Check sheet for the modelled part. Datum: model origin and axes. Units: mm. Face numbers are marked on the shaded views. A direction names the side the tool comes from. Coordinates: 2 decimals unless noted, no trailing zeros. Loops run counter-clockwise (first coordinate to the right, second up) from the corner with the lowest first, then second, coordinate; pieces in that order, holes last. Notation, with made-up numbers: (61.25, -14.75) - (117.25, -14.75) arc R20 cw to (117.25, 22.25) - close; hole circle Ø10 at (-15.5, -23). An arc over 180 degrees is marked (long way). Write each question's results on one line, items separated by ' | '. Start each with the question number.
1. Gauge pin test, flat ends, axial feed: P1, Ø12, axis at y = 31, z = 2.5, coming from the -X side; P2, Ø4, axis at y = 26, z = -18.5, coming from the +X side; P3, Ø6, axis at y = 20, z = 18.5, coming from the +X side; P4, Ø1.5, axis at x = -38.5, y = 20.5, coming from the -Z side. Record the tip position at first contact, or that the pin passes through.
2. Draft check along Z on the marked faces 6, 7, 8 and 9. Enter one of: released by +Z, released by -Z, zero draft, split by the parting line, or undercut.
3. Tool access check on the marked faces 1, 2, 3, 4 and 5. Record the directions out of +Z, -Z, +X, -X, +Y, -Y that give a thin tool (end or side, any length) a straight path to the whole face; none if there is none.
4. Cross-section at C-C (x = -33). Give the number of separate pieces and of enclosed holes in the cut face, and give its area (3 significant figures).
5. Cross-section at A-A (z = -33.5). Record the cut outline in (x, y).
6. Thickness scan on line 1 (Z direction, x = -29.5, y = 29); line 2 (Z direction, x = -17.5, y = 22); line 3 (Y direction, x = -31.5, z = -1). Record the ranges inside material, lowest first. Write a range as [from, to].
7. Cross-section at D-D (z = -15). Record the cut outline in (x, y), and give its area (3 significant figures).
8. Cross-section at B-B (y = 14). Record the cut outline in (x, z), and give its area (3 significant figures).
```python
from build123d import *

# Parameters (mm, degrees)
F0_R      = 8.5
F1_DEPTH  = 32
F4_DEPTH  = 32.4
F5_SIZE   = 1
F6_R      = 15
F7_DEPTH  = 16
F8_R      = 8.5
F9_DEPTH  = 32
F10_SIZE  = 1
F13_DEPTH = 46.1
F15_R     = 6.055959
F16_DEPTH = 53.1


with BuildPart() as f1:
    # F0 (on Top) → F1 (new body)
    with BuildSketch(Plane.XY):
        with Locations((-31.744916, 24.020635)):
            Circle(F0_R)
    extrude(amount=F1_DEPTH)

    # F3 (on offset) → F4 (cut)
    with BuildSketch(Plane.XZ.offset(-33)):
        with BuildLine():
            ThreePointArc((-28.736681, 21.964274), (-31.682465, 24.910059), (-34.62825, 21.964274))
            Line((-34.62825, 21.964274), (-34.62825, 9.964274))
            ThreePointArc((-34.62825, 9.964274), (-31.682465, 7.01849), (-28.736681, 9.964274))
            Line((-28.736681, 9.964274), (-28.736681, 21.964274))
        make_face()
    extrude(amount=F4_DEPTH, mode=Mode.SUBTRACT)

    # F5
    f5_edges = [f1.edges().sort_by_distance(p)[0] for p in [
        (-40.244916, 24.020635, 32),
    ]]
    chamfer(f5_edges, length=F5_SIZE)

    # F6 (on face) → F7 (join)
    with BuildSketch(Plane(origin=(0, 0, 0), x_dir=(1, 0, 0), z_dir=(0, 0, -1))):
        with Locations((-31.744916, -24.020635)):
            Circle(F6_R)
    extrude(amount=F7_DEPTH)

    # F8 (on face) → F9 (join)
    with BuildSketch(Plane(origin=(0, 0, -16), x_dir=(1, 0, 0), z_dir=(0, 0, -1))):
        with Locations((-31.744916, -24.020635)):
            Circle(F8_R)
    extrude(amount=F9_DEPTH)

    # F10
    f10_edges = [f1.edges().sort_by_distance(p)[0] for p in [
        (-40.244916, 24.020635, -48),
    ]]
    chamfer(f10_edges, length=F10_SIZE)

    # F12 (on offset) → F13 (cut)
    with BuildSketch(Plane.XZ.offset(-35.2)):
        with BuildLine():
            Line((-28.785402, -37.644354), (-28.785402, -25.994403))
            ThreePointArc((-28.785402, -25.994403), (-31.785402, -22.994403), (-34.785402, -25.994403))
            Line((-34.785402, -25.994403), (-34.785402, -37.644354))
            ThreePointArc((-34.785402, -37.644354), (-31.785402, -40.644354), (-28.785402, -37.644354))
        make_face()
    extrude(amount=F13_DEPTH, mode=Mode.SUBTRACT)

    # F15 (on offset) → F16 (cut)
    with BuildSketch(Plane.XZ.offset(-41.4)):
        with Locations((-31.784016, -7.985172)):
            Circle(F15_R)
    extrude(amount=F16_DEPTH, mode=Mode.SUBTRACT)


solid = f1.part
```
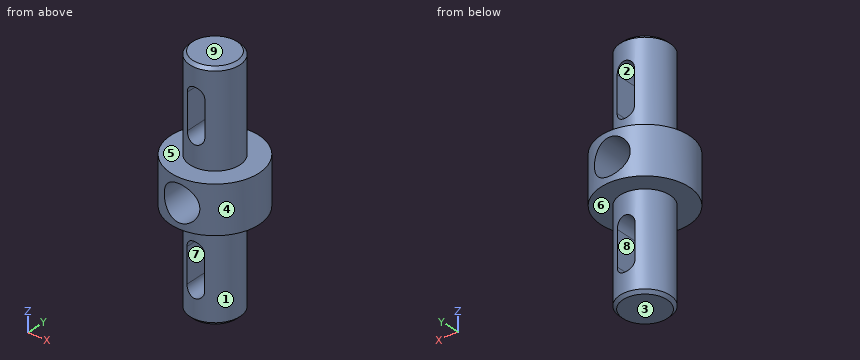
Established:
1) P1: x = -46.67 | P2: x = -23.24 | P3: x = -23.31 | P4: z = -48
2) face 6: released by -Z | face 7: undercut | face 8: undercut | face 9: released by +Z
3) face 1: -Z | face 2: +Y, -Y | face 3: -Z, +X, -X, +Y, -Y | face 4: +Z, -Z | face 5: +Z
4) separate pieces: 4 | enclosed holes: 0 | area: 619 mm^2
5) outline: (-34.79, 16.08) - (-34.79, 31.96) arc R8.5 ccw to start; (-28.79, 16.05) arc R8.5 ccw to (-28.79, 31.99) - close
6) line 1: [-48, -39.59], [-24.05, -13.59], [-2.38, 7.99], [23.94, 32] | line 2: [-16, 0] | line 3: [9.02, 39.02]
7) outline: circle Ø30 at (-31.74, 24.02) | area: 707 mm^2
8) outline: (-42.91, -16) - (-20.58, -16) - (-20.58, 0) - (-42.91, 0) - close; hole circle Ø12.11 at (-31.78, -7.99) | area: 242 mm^2
